CAD build for the part. Positions are in the model's coordinates, mm. Coordinates: 2 decimals unless noted, no trailing zeros. Write each loop counter-clockwise with the first axis right and the second up, starting at its lowest first coordinate (ties: lowest second). Pieces come first, ordered by that corner, then holes. Notation, with made-up numbers: (49.5, 85.25) - (62.5, 85.25) arc R21 cw to (62.5, 108.25) - close; hole circle Ø8 at (84.5, 77.25). An arc over 180 degrees is marked (long way). Answer in a Markdown table with one row per item. Add a question column.
Q1. Pin check, flat tips, straight feed: pin 1 (1.8 mm diameter, centred on y = 11.5, z = 50, fed in from -X); pin 2 (5.5 mm diameter, centred on x = -476, z = 102, fed in from +Y). Stop position of each tip, or through.
Q2. Drill centre lines: line 1 along Z through (x, y) = (-484.5, 12); line 2 along Z through (x, y) = (-478, 11); line 3 along Z through (x, y) = (-476, 17.25). Where is each one in solid material? Low to high. Write a range as from..to.
Q3. Band-saw the part on A-A (z = 102). List the corners of the cut face in (x, y).
Q4. Band-saw the part on B-B (z = 50). List the corners of the cut face in (x, y), and give its area (3 significant figures).
Q5. Band-saw the part on C-C (y = 12.75). List the corners of the cut face in (x, z).
Q6. Two-plate mould, pull along Y, no slides. Class faces 1 (the flat face through (-476, 12, 50)), 2 (the flat face through (-476, 24, 75)), 3 (the flat face through (-500, 12, 75)), 4 (the cylindrical face through (-488, 12, 53)): +Y half, -Y half, draft (parallel to the pull), parting line (faces both ways), or undercut.
```python
from build123d import *

# Parameters (mm, degrees)
SKETCH071_W             = 48
SKETCH071_H             = 24
PAD039_DEPTH            = 100
SKETCH069_R             = 3
POCKET031_DEPTH         = 24
SKETCH070_R             = 3
POCKET030_DEPTH         = 24.001
BODY045_PLACEMENT_ANGLE = 180


with BuildPart() as part:
    # Sketch071 → Pad039 (new body)
    with BuildSketch(Plane.XY):
        with Locations((24, 12)):
            Rectangle(SKETCH071_W, SKETCH071_H)
    extrude(amount=PAD039_DEPTH)

    # Sketch069 (on Face2 of Pad039) → Pocket031 (cut)
    with BuildSketch(Plane.YZ.offset(48)):
        with Locations((12, 24)):
            Circle(SKETCH069_R)
    extrude(amount=-POCKET031_DEPTH, mode=Mode.SUBTRACT)

    # Sketch070 (on Face1 of Pocket031) → Pocket030 (cut, through all)
    with BuildSketch(Plane.XZ):
        with Locations((24, 76)):
            Circle(SKETCH070_R)
    extrude(amount=-POCKET030_DEPTH, mode=Mode.SUBTRACT)


with BuildPart() as part_1:
    # Body045 placement: moved
    add(part.part.moved(Location((-452, 24, 26))).rotate(Axis((-452, 24, 26), (0, 0, 1)), BODY045_PLACEMENT_ANGLE))


solid = part_1.part
```
Checked values:
| question | item | result |
|---|---|---|
| 1 | pin 1 | stops at x = -476 |
| 1 | pin 2 | passes through |
| 2 | line 1 | z = 26..47, 53..126 |
| 2 | line 2 | z = 26..47.17, 52.83..99.76, 104.24..126 |
| 2 | line 3 | z = 26..99, 105..126 |
| 3 | outline | (-500, 0) - (-479, 0) - (-479, 24) - (-500, 24) - close; (-473, 0) - (-452, 0) - (-452, 24) - (-473, 24) - close |
| 4 | outline | (-500, 0) - (-452, 0) - (-452, 24) - (-500, 24) - (-500, 15) - (-476, 15) - (-476, 9) - (-500, 9) - close |
| 4 | area | 1,010 mm² |
| 5 | outline | (-500, 26) - (-452, 26) - (-452, 126) - (-500, 126) - (-500, 52.9) - (-476, 52.9) - (-476, 47.1) - (-500, 47.1) - close; hole circle Ø6 at (-476, 102) |
| 6 | face 1 | undercut |
| 6 | face 2 | +Y half |
| 6 | face 3 | draft |
| 6 | face 4 | undercut |
